from build123d import *

# Parameters (mm, degrees)
SKETCH_2_R      = 20
SKETCH_2_R_2    = 2
EXTRUDE_1_DEPTH = 25


with BuildPart() as part:
    # 草图2 → 凸台-拉伸1 (new body)
    with BuildSketch(Plane(origin=(0, 0, 0), x_dir=(1, 0, 0), z_dir=(0, 1, 0))):
        Circle(SKETCH_2_R)
        with Locations((-5, 5)):
            Circle(SKETCH_2_R_2, mode=Mode.SUBTRACT)
        with Locations((5, 5)):
            Circle(SKETCH_2_R_2, mode=Mode.SUBTRACT)
        with Locations((5, -5)):
            Circle(SKETCH_2_R_2, mode=Mode.SUBTRACT)
        with Locations((-5, -5)):
            Circle(SKETCH_2_R_2, mode=Mode.SUBTRACT)
        with BuildLine():
            Line((-8.445719569, 7.031506006), (-13.415371808, 12.001158246))
            ThreePointArc((-13.415371808, 12.001158246), (-18, 0), (-13.415371808, -12.001158246))
            Line((-13.415371808, -12.001158246), (-8.445719569, -7.031506006))
            ThreePointArc((-8.445719569, -7.031506006), (-8.69551813, -3.469266271), (-6, -1.127016654))
            Line((-6, -1.127016654), (-6, 1.127016654))
            ThreePointArc((-6, 1.127016654), (-8.69551813, 3.469266271), (-8.445719569, 7.031506006))
        make_face(mode=Mode.SUBTRACT)
        with BuildLine():
            Line((-12.001158246, 13.415371808), (-7.031506006, 8.445719569))
            ThreePointArc((-7.031506006, 8.445719569), (-3.469266271, 8.69551813), (-1.127016654, 6))
            Line((-1.127016654, 6), (1.127016654, 6))
            ThreePointArc((1.127016654, 6), (3.469266271, 8.69551813), (7.031506006, 8.445719569))
            Line((7.031506006, 8.445719569), (12.001158246, 13.415371808))
            ThreePointArc((12.001158246, 13.415371808), (0, 18), (-12.001158246, 13.415371808))
        make_face(mode=Mode.SUBTRACT)
        with BuildLine():
            Line((13.415371808, 12.001158246), (8.445719569, 7.031506006))
            ThreePointArc((8.445719569, 7.031506006), (8.69551813, 3.469266271), (6, 1.127016654))
            Line((6, 1.127016654), (6, -1.127016654))
            ThreePointArc((6, -1.127016654), (8.69551813, -3.469266271), (8.445719569, -7.031506006))
            Line((8.445719569, -7.031506006), (13.415371808, -12.001158246))
            ThreePointArc((13.415371808, -12.001158246), (18, 0), (13.415371808, 12.001158246))
        make_face(mode=Mode.SUBTRACT)
        with BuildLine():
            Line((12.001158246, -13.415371808), (7.031506006, -8.445719569))
            ThreePointArc((7.031506006, -8.445719569), (3.469266271, -8.69551813), (1.127016654, -6))
            Line((1.127016654, -6), (-1.127016654, -6))
            ThreePointArc((-1.127016654, -6), (-3.469266271, -8.69551813), (-7.031506006, -8.445719569))
            Line((-7.031506006, -8.445719569), (-12.001158246, -13.415371808))
            ThreePointArc((-12.001158246, -13.415371808), (0, -18), (12.001158246, -13.415371808))
        make_face(mode=Mode.SUBTRACT)
        with BuildLine():
            Line((-1.127016654, 4), (1.127016654, 4))
            ThreePointArc((1.127016654, 4), (2.171572875, 2.171572875), (4, 1.127016654))
            Line((4, 1.127016654), (4, -1.127016654))
            ThreePointArc((4, -1.127016654), (2.171572875, -2.171572875), (1.127016654, -4))
            Line((1.127016654, -4), (-1.127016654, -4))
            ThreePointArc((-1.127016654, -4), (-2.171572875, -2.171572875), (-4, -1.127016654))
            Line((-4, -1.127016654), (-4, 1.127016654))
            ThreePointArc((-4, 1.127016654), (-2.171572875, 2.171572875), (-1.127016654, 4))
        make_face(mode=Mode.SUBTRACT)
    extrude(amount=EXTRUDE_1_DEPTH)


solid = part.part
Model file for the job. Use its own axes, mm. Coordinates: 2 decimals unless noted, no trailing zeros. Loops run counter-clockwise (first coordinate to the right, second up) from the corner with the lowest first, then second, coordinate; pieces in that order, holes last. Notation, with made-up numbers: (67.25, 87) -> (107.25, 87) arc R10 cw to (107.25, 93) -> close; hole circle Ø4 at (17, 77.25). An arc over 180 degrees is marked (long way). Use one line per item in the form item = value. Start each with the question number.
(1) Cut at D-D on x = 15. Give the cut face in (y, z).
(2) Cut at A-A on x = -4.5. Give the cut face in (y, z).
(3) Cut at C-C on z = -17. Give the cut face in (x, y).
(4) Cut at B-B on z = -5. Give the cut face in (x, y), and give its area (3 significant figures).
(5) Pull direction X, two halves, no side cores. Call faces 1 (the cylindrical face through (3.422, 12.325, -8.675)), 2 (the flat face through (6, 12, 0)), 3 (the flat face through (-3, 0, 3)): pulls with the +X half, pulls with the -X half, needs draft (parallel to the pull), parting line crosses it, or undercut.
(6) Probe probe 1 along Z at (x, y) = (5, 6); probe 2 along Z at (x, y) = (1, 5.5). List the from-to ranges inside material, lowest first. Write a range as from..to.
(7) Flat gauge pins, fed straight in: pin 1 (12 mm diameter, centred on x = 6.5, y = 13.5, fed in from +Z); pin 2 (1.8 mm diameter, centred on x = 0.5, y = 11, fed in from -Z); pin 3 (12 mm diameter, centred on x = -8.5, y = 19.5, fed in from +Z); pin 4 (2.5 mm diameter, centred on x = -5, z = -5, fed in from -Y). Where does each tip first touch, or does it go through?
Values:
q1.outline = (0, -13.23) -> (25, -13.23) -> (25, -9.95) -> (0, -9.95) -> close; (0, 9.95) -> (25, 9.95) -> (25, 13.23) -> (0, 13.23) -> close
q2.outline = (0, -19.49) -> (25, -19.49) -> (25, -17.43) -> (0, -17.43) -> close; (0, -8.97) -> (25, -8.97) -> (25, -6.94) -> (0, -6.94) -> close; (0, -3.06) -> (25, -3.06) -> (25, 3.06) -> (0, 3.06) -> close; (0, 6.94) -> (25, 6.94) -> (25, 8.97) -> (0, 8.97) -> close; (0, 17.43) -> (25, 17.43) -> (25, 19.49) -> (0, 19.49) -> close
q3.outline = (-10.54, 0) -> (-5.92, 0) -> (-5.92, 25) -> (-10.54, 25) -> close; (5.92, 0) -> (10.54, 0) -> (10.54, 25) -> (5.92, 25) -> close
q4.outline = (-19.36, 0) -> (-17.29, 0) -> (-17.29, 25) -> (-19.36, 25) -> close; (-9, 0) -> (-7, 0) -> (-7, 25) -> (-9, 25) -> close; (-3, 0) -> (3, 0) -> (3, 25) -> (-3, 25) -> close; (7, 0) -> (9, 0) -> (9, 25) -> (7, 25) -> close; (17.29, 0) -> (19.36, 0) -> (19.36, 25) -> (17.29, 25) -> close
q4.area = 354 mm2
q5.face_1 = undercut
q5.face_2 = undercut
q5.face_3 = needs draft
q6.probe_1 = -19.36..-17.29, -9..-7, -3..3, 7..9, 17.29..19.36
q6.probe_2 = -19.97..-17.97, -6..-4, 4..6, 17.97..19.97
q7.pin_1 = 19.99
q7.pin_2 = -20
q7.pin_3 = 19.84
q7.pin_4 = through
